Design review of the part shown in the three views and the two pictorial views. Dimensions are in mm from the part's minimum x, y and z. Coordinates: 2 decimals unless noted, no trailing zeros. Loops run counter-clockwise (first coordinate to the right, second up) from the corner with the lowest first, then second, coordinate; pieces in that order, holes last. Notation, with made-up numbers: (78, 27.5) -> (96, 27.5) arc R16 cw to (96, 35.5) -> close; hole circle Ø3 at (83, 76.5). An arc over 180 degrees is marked (long way). One line per item, written item: value. Start each with the question number.
1. Add section B-B on x = 69. Write out the cut boundary in (y, z).
2. Add section D-D on x = 132. Write out the cut boundary in (y, z).
3. For probe 1 along Y at (x, z) = (69, 2.25); probe 2 along Y at (x, z) = (15, 0.6); probe 3 along Y at (x, z) = (98.5, 0.85), list the stretches that pass through material, from the lowest coordinate up.
4. Insertion check: pin 1 (1.5 mm diameter, centred on x = 62.5, z = 3, fed in from -Y); pin 2 (1.5 mm diameter, centred on x = 40.5, z = 1.5, fed in from +Y). Each pin has a flat end and moves straight along its axis. Give the tip position at first contact, or say it passes through.
5. Add section C-C on z = 2.65. Write out the cut boundary in (x, y), plus the area to 3 significant figures.
6. Add section A-A on y = 15. Write out the cut boundary in (x, z).
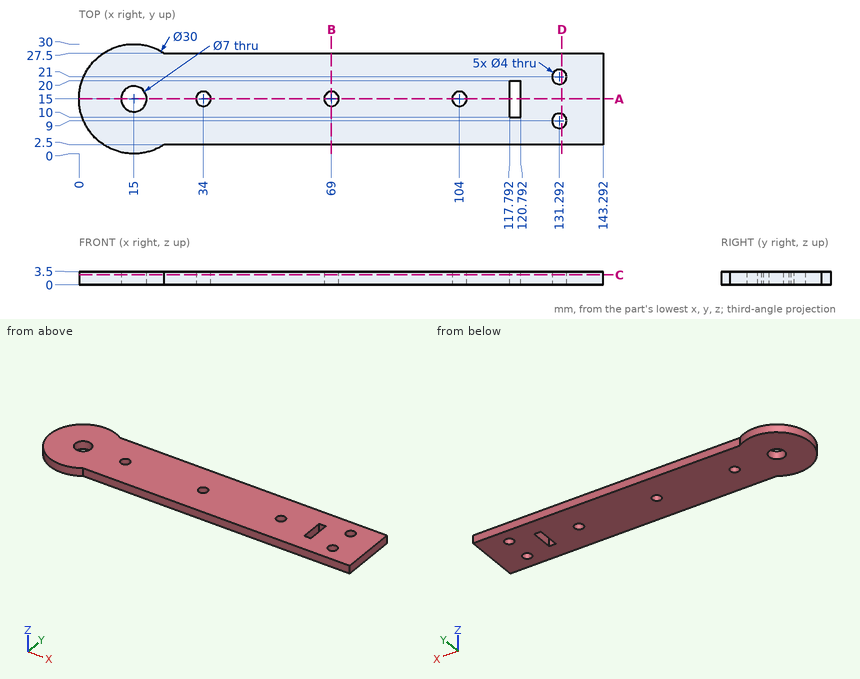
Worked answers:
1. outline: (2.5, 0) -> (13, 0) -> (13, 3.5) -> (2.5, 3.5) -> close; (17, 0) -> (27.5, 0) -> (27.5, 3.5) -> (17, 3.5) -> close
2. outline: (2.5, 0) -> (7.13, 0) -> (7.13, 3.5) -> (2.5, 3.5) -> close; (10.87, 0) -> (19.13, 0) -> (19.13, 3.5) -> (10.87, 3.5) -> close; (22.87, 0) -> (27.5, 0) -> (27.5, 3.5) -> (22.87, 3.5) -> close
3. probe 1: y = 2.5 to 13, 17 to 27.5
3. probe 2: y = 0 to 11.5, 18.5 to 30
3. probe 3: y = 2.5 to 27.5
4. pin 1: stops at y = 2.5
4. pin 2: stops at y = 27.5
5. outline: (23.29, 2.5) -> (143.29, 2.5) -> (143.29, 27.5) -> (23.29, 27.5) arc R15 ccw (long way) to start; hole circle Ø7 at (15, 15); hole circle Ø4 at (34, 15); hole circle Ø4 at (69, 15); hole circle Ø4 at (104, 15); hole (117.79, 10) -> (120.79, 10) -> (120.79, 20) -> (117.79, 20) -> close; hole circle Ø4 at (131.29, 9); hole circle Ø4 at (131.29, 21)
5. area: 3,460 mm²
6. outline: (0, 0) -> (11.5, 0) -> (11.5, 3.5) -> (0, 3.5) -> close; (18.5, 0) -> (32, 0) -> (32, 3.5) -> (18.5, 3.5) -> close; (36, 0) -> (67, 0) -> (67, 3.5) -> (36, 3.5) -> close; (71, 0) -> (102, 0) -> (102, 3.5) -> (71, 3.5) -> close; (106, 0) -> (117.79, 0) -> (117.79, 3.5) -> (106, 3.5) -> close; (120.79, 0) -> (143.29, 0) -> (143.29, 3.5) -> (120.79, 3.5) -> close
